Input: part model. Units: mm. Frame: model coordinates. Face numbers are marked on the shaded views. A direction names the side the tool comes from. Coordinates: 2 decimals unless noted, no trailing zeros. Write each loop counter-clockwise with the first axis right and the second up, starting at its lowest first coordinate (ties: lowest second). Pieces come first, ordered by that corner, then holes. Notation, with made-up numbers: M 44.25,62 L 70.25,62 A36 ccw 70.25,100 Z; hole C 48.5,27.25 d5. An arc over 180 degrees is marked long. Answer as a JSON object with one key per item and string values. Group by question number.
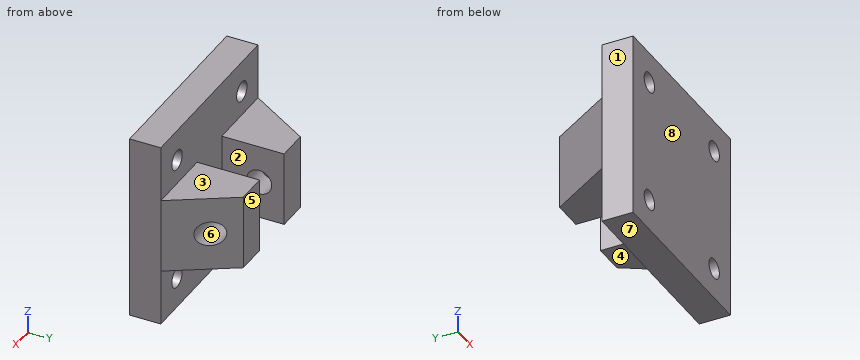
from build123d import *

# Parameters (mm, degrees)
SKETCH1_W                = 30
SKETCH1_H                = 30
BOSS_EXTRUDE1_DEPTH      = 5
BOSS_EXTRUDE2_DEPTH      = 6
BOSS_EXTRUDE2_DEPTH_BACK = 6
M3_CLEARANCE_HOLE1_D     = 3.2
CUT_EXTRUDE1_DEPTH       = 26.980762114
CUT_EXTRUDE1_DEPTH_BACK  = 8
SKETCH5_R                = 2


with BuildPart() as part:
    # Sketch1 → Boss-Extrude1 (new body)
    with BuildSketch(Plane(origin=(0, 0, 0), x_dir=(1, 0, 0), z_dir=(0, 1, 0))):
        Rectangle(SKETCH1_W, SKETCH1_H)
    extrude(amount=BOSS_EXTRUDE1_DEPTH)

    # Sketch2 → Boss-Extrude2 (add, two sides: drawn at the far end of the back side and taken through both)
    with BuildSketch(Plane.XY.offset(-BOSS_EXTRUDE2_DEPTH_BACK)):
        Polygon((15, 0), (-15, 0), (-15, 5), (-8.81, 15), (-3.81, 15), (-3.81, 5), (3.81, 5), (3.81, 15), (8.81, 15), (15, 5), align=None)
    extrude(amount=BOSS_EXTRUDE2_DEPTH + BOSS_EXTRUDE2_DEPTH_BACK)

    # M3 Clearance Hole1 (through all)
    with Locations(Plane(origin=(0, 5, 0), x_dir=(1, 0, 0), z_dir=(0, 1, 0))):
        with Locations((-10, 10), (10, 10), (10, -10), (-10, -10)):
            Hole(M3_CLEARANCE_HOLE1_D / 2)

    # Sketch5 → Cut-Extrude1 (cut, two sides: drawn at the far end of the back side and taken through both)
    with BuildSketch(Plane(origin=(0, 0, 0), x_dir=(0, 0, -1), z_dir=(1, 0, 0)).offset(-CUT_EXTRUDE1_DEPTH_BACK)):
        with Locations(Location((0, 11, 0), (0, 0, 270))):
            Circle(SKETCH5_R)
    extrude(amount=CUT_EXTRUDE1_DEPTH + CUT_EXTRUDE1_DEPTH_BACK, mode=Mode.SUBTRACT)


solid = part.part
Q1. Draft query along Y for the marked faces 5, 6, 7 and 8. Return one class per face: released by +Y, released by -Y, zero draft, split by the parting line, or undercut.
Q2. Line query: line 1 (X direction, y = 2.3, z = 10); line 2 (Y direction, x = 11.5, z = 9). Output: solid intervals per line, ascending. Write a range as from..to.
Q3. Pin query (flat end, axial travel): pin 1 Ø1.2 at (y, z) = (10.5, 0) entering from +X; pin 2 Ø4 at (y, z) = (8.5, 1) entering from -X; pin 3 Ø3 at (x, y) = (-8, 11.5) entering from -Z; pin 4 Ø1 at (x, z) = (5.5, -8.5) entering from -Y. Return the tip coordinate at first contact, or that it passes through.
Q4. Section D-D, the plane y = 13.5. Return the cut outline in (x, z).
Q5. Section C-C, the plane z = -10. Return the cut outline in (x, y), and give its area (3 significant figures).
Q6. Section B-B, the plane y = 10.5. Return the cut outline in (x, z), and give its area (3 significant figures).
Q7. Access query for the marked faces 1, 2, 3 and 4. Directions: +Z, -Z, +X, -X, +Y, -Y. A direction counts if a zero-diameter tool reaches every point of the face in a straight line with its end or side. Return the directions, or none.
Q8. Section A-A, the plane x = 8. Return the cut outline in (y, z).
Filled in:
{
 "1": {"face 5": "released by +Y", "face 6": "undercut", "face 7": "zero draft", "face 8": "released by -Y"},
 "2": {"line 1": "-15..-11.6, -8.4..8.4, 11.6..15", "line 2": "0..5"},
 "3": {"pin 1": "x = -8", "pin 2": "x = -14.07", "pin 3": "z = -6", "pin 4": "y = 0"},
 "4": {"outline": "M -9.74,-6 L -3.81,-6 L -3.81,6 L -9.74,6 Z; M 3.81,-6 L 9.74,-6 L 9.74,6 L 3.81,6 Z"},
 "5": {"outline": "M -15,0 L -11.6,0 L -11.6,5 L -15,5 Z; M -8.4,0 L 8.4,0 L 8.4,5 L -8.4,5 Z; M 11.6,0 L 15,0 L 15,5 L 11.6,5 Z", "area": "118 mm^2"},
 "6": {"outline": "M -11.6,-6 L -3.81,-6 L -3.81,-1.94 L -8,-1.94 L -8,1.94 L -3.81,1.94 L -3.81,6 L -11.6,6 Z; M 3.81,-6 L 11.6,-6 L 11.6,-1.94 L 3.81,-1.94 Z; M 3.81,1.94 L 11.6,1.94 L 11.6,6 L 3.81,6 Z", "area": "140 mm^2"},
 "7": {"face 1": "+Z, -Z, -X, +Y, -Y", "face 2": "+Z, -Z, +Y", "face 3": "+Z, +X, -X, +Y", "face 4": "-Z, +X, -X, +Y"},
 "8": {"outline": "M 0,-15 L 5,-15 L 5,-6 L 15,-6 L 15,6 L 5,6 L 5,15 L 0,15 Z; hole C 11,0 d4"}
}
